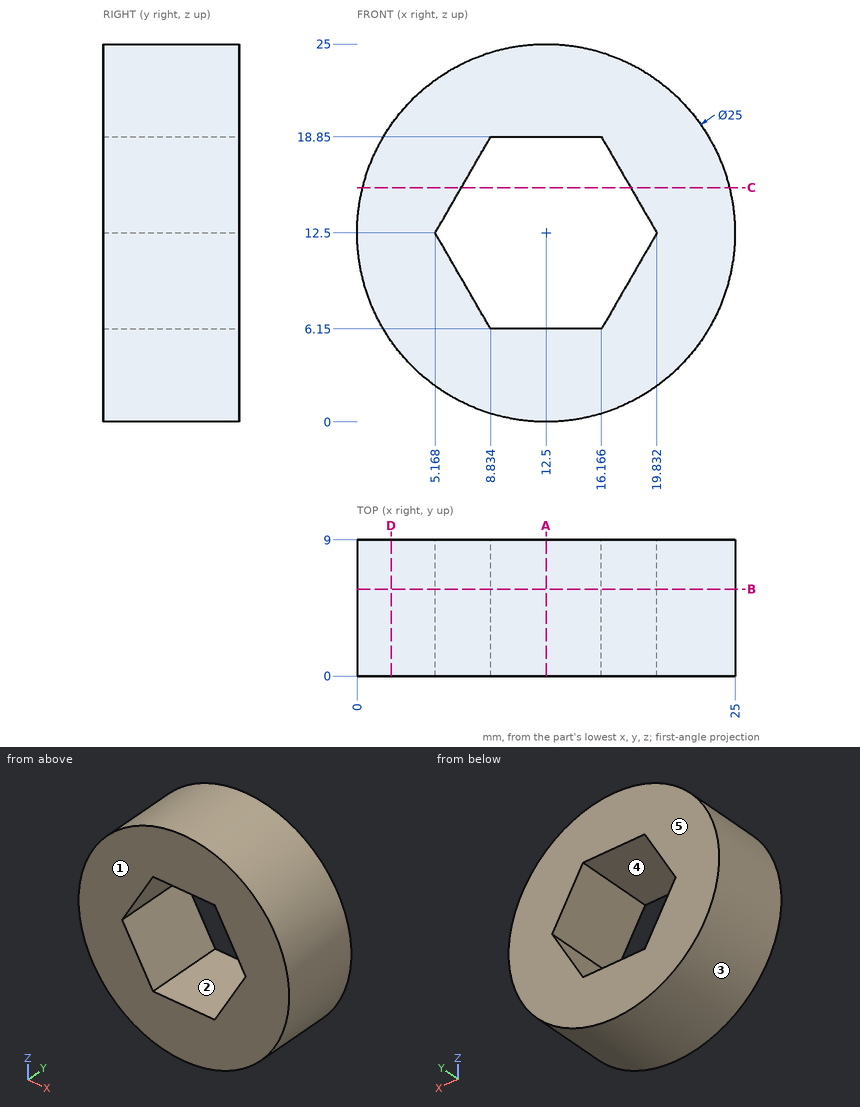
Source: three-view drawing plus pictorial views. Frame: mm from the lowest corner of the part. A direction names the side the tool comes from. Give positions to 0.01 mm unless a question says otherwise; leave off trailing zeros. Loops run counter-clockwise (first coordinate to the right, second up) from the corner with the lowest first, then second, coordinate; pieces in that order, holes last. Notation, with made-up numbers: (52.25, 40.25) -> (109.25, 40.25) arc R25 cw to (109.25, 62.25) -> close; hole circle Ø3 at (-20.5, 74). An arc over 180 degrees is marked (long way). Put each result on its own line as item: value. Start each with the question number.
1) Cut plane C-C (z = 15.5). Return loops of the section in (x, y) (1 decimal), then the cut area to 3 significant figures.
2) Material intervals for probe 1 along X at (y, z) = (8.25, 18.25); probe 2 along Z at (x, y) = (18.75, 3) (1 decimal); probe 3 along X at (y, z) = (5.5, 16), sorted ascending.
3) Draft query along Z for the marked faces 1, 2 and 3. Return one class per face: released by +Z, released by -Z, zero draft, split by the parting line, or undercut.
4) Reachability of the marked faces 4 and 5 from +Z, -Z, +X, -X, +Y, -Y: full face, straight path, thin tool, end or side. Return the list, or none.
5) Cut plane D-D (x = 2.25). Return loops of the section in (y, z) (1 decimal), then the cut area to 3 significant figures.
6) Cut plane A-A (x = 12.5). Return loops of the section in (y, z).
7) Contact query for flat-ended pins moving along their axis: P1, Ø1, axis at x = 11, y = 1, coming from the -Z side; P2, Ø1, axis at y = 3, z = 10.5, coming from the +X side; P3, Ø1, axis at x = 21.5, y = 1, coming from the -Z side (1 decimal); P4, Ø1.5, axis at x = 8, z = 13, coming from the -Y side. Output: stop coordinate, or through.
8) Cut plane B-B (y = 5.75). Return loops of the section in (x, z), then the cut area to 3 significant figures.
Results are:
1. outline: (0.4, 0) -> (6.9, 0) -> (6.9, 9) -> (0.4, 9) -> close; (18.1, 0) -> (24.6, 0) -> (24.6, 9) -> (18.1, 9) -> close
1. area: 118 mm2
2. probe 1: x = 1.4 to 8.49, 16.51 to 23.6
2. probe 2: z = 1.7 to 10.6, 14.4 to 23.3
2. probe 3: x = 0.5 to 7.19, 17.81 to 24.5
3. face 1: zero draft
3. face 2: undercut
3. face 3: split by the parting line
4. face 4: +Y, -Y
4. face 5: +Z, -Z, +X, -X, +Y
5. outline: (0, 5.3) -> (9, 5.3) -> (9, 19.7) -> (0, 19.7) -> close
5. area: 129 mm2
6. outline: (0, 0) -> (9, 0) -> (9, 6.15) -> (0, 6.15) -> close; (0, 18.85) -> (9, 18.85) -> (9, 25) -> (0, 25) -> close
7. P1: stops at z = 0.04
7. P2: stops at x = 24.91
7. P3: stops at z = 3.3
7. P4: passes through
8. outline: circle Ø25 at (12.5, 12.5); hole (5.17, 12.5) -> (8.83, 6.15) -> (16.17, 6.15) -> (19.83, 12.5) -> (16.17, 18.85) -> (8.83, 18.85) -> close
8. area: 351 mm2
